Drawing for the job (mm, zero at the part's lowest x, y, z). A direction names the side the tool comes from. Round coordinates to 2 decimals unless told otherwise and drop trailing zeros. Write each loop counter-clockwise with the first axis right and the second up, starting at its lowest first coordinate (ties: lowest second). Pieces come first, ordered by that corner, then holes. Notation, with made-up numbers: M 35.25,13 L 86.25,13 A15 cw 86.25,20 Z; hole C 0.25,7.5 d3. An arc over 180 degrees is marked long. Use a Markdown table: item, result.
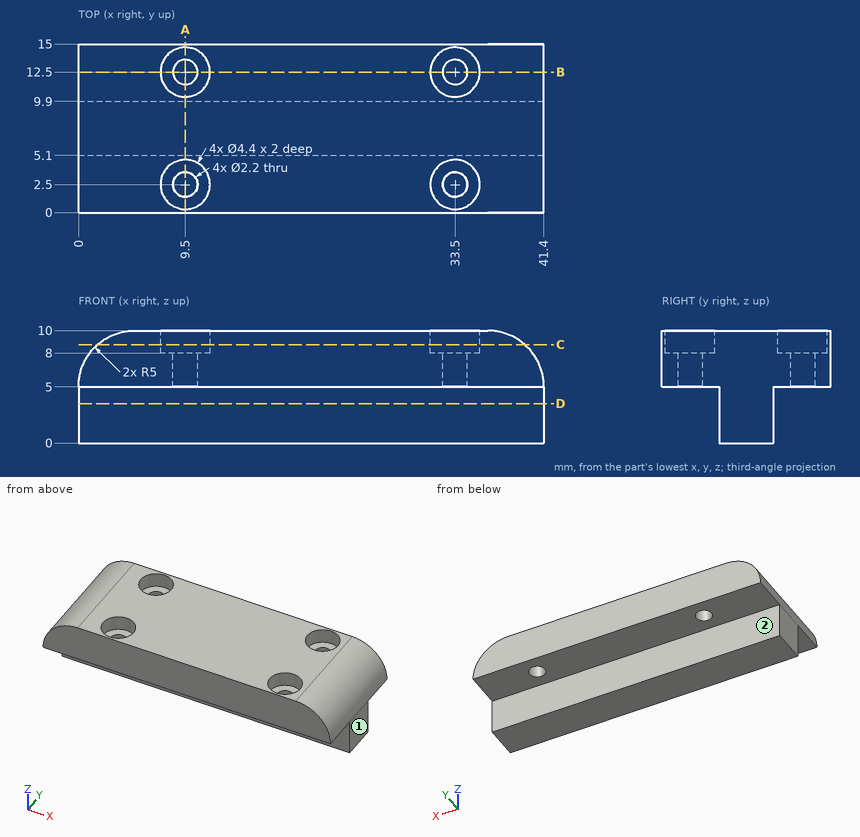
Q1. Drop flat-ended pins along their axis: P1, Ø2, axis at y = 13, z = 9, coming from the -X side; P2, Ø3.5, axis at x = 33.5, y = 2.5, coming from the +Z side; P3, Ø2.5, axis at x = 17.5, y = 12, coming from the -Z side; P4, Ø1.3, axis at x = 9.5, y = 12.5, coming from the -Z side. Give the stop position or say it passes through.
Response values:
| item | result |
|---|---|
| P1 | stops at x = 1 |
| P2 | stops at z = 8 |
| P3 | stops at z = 5 |
| P4 | passes through |
Q2. Cut at D-D on z = 3.5. Give the cut face in (x, y), and give its area (3 significant figures).
Response values:
| item | result |
|---|---|
| outline | M 0,5.1 L 41.4,5.1 L 41.4,9.9 L 0,9.9 Z |
| area | 199 mm2 |
Q3. Which spindle directions (+Z, -Z, +X, -X, +Y, -Y) get a long thin tool onto all of the face, cutting with end or side? Do the marked faces 1 and 2. Say none if no direction does.
Response values:
| item | result |
|---|---|
| face 1 | +Z, -Z, +X, +Y, -Y |
| face 2 | -Z, +X, -X, +Y |
Q4. Cut at A-A on x = 9.5. Give the cut face in (y, z), and give its area (3 significant figures).
Response values:
| item | result |
|---|---|
| outline | M 0,5 L 1.4,5 L 1.4,8 L 0.3,8 L 0.3,10 L 0,10 Z; M 3.6,5 L 5.1,5 L 5.1,0 L 9.9,0 L 9.9,5 L 11.4,5 L 11.4,8 L 10.3,8 L 10.3,10 L 4.7,10 L 4.7,8 L 3.6,8 Z; M 13.6,5 L 15,5 L 15,10 L 14.7,10 L 14.7,8 L 13.6,8 Z |
| area | 68.2 mm2 |
Q5. Cut at C-C on z = 8.75. Give the cut face in (x, y).
Response values:
| item | result |
|---|---|
| outline | M 1.69,0 L 39.71,0 L 39.71,15 L 1.69,15 Z; hole C 9.5,2.5 d4.4; hole C 9.5,12.5 d4.4; hole C 33.5,2.5 d4.4; hole C 33.5,12.5 d4.4 |
Q6. Drill centre lines: L1, parallel to Y at x = 33.5, z = 6.65; L2, parallel to Y at x = 9.5, z = 9.45; L3, parallel to Z at x = 29.5, y = 10.5. Where is each one in solid material? Low to high.
Response values:
| item | result |
|---|---|
| L1 | y = 0 to 1.4, 3.6 to 11.4, 13.6 to 15 |
| L2 | y = 0 to 0.3, 4.7 to 10.3, 14.7 to 15 |
| L3 | z = 5 to 10 |
Q7. Cut at B-B on y = 12.5. Count the separate pieces of the cut face and the enclosed holes in it, and give its area (3 significant figures).
Response values:
| item | result |
|---|---|
| separate pieces | 3 |
| enclosed holes | 0 |
| area | 165 mm2 |
